Could you check a few things on this model? Use its own coordinates, in mm. A direction names the side the tool comes from. Give positions to 0.01 mm unless a question says otherwise; leave off trailing zeros. Loops run counter-clockwise (first coordinate to the right, second up) from the corner with the lowest first, then second, coordinate; pieces in that order, holes last.
1. Imagine slicing it at A-A (z = -29.5). List the corners of the cut face in (x, y) for me.
2. For faces 4 (the cylindrical face through (-0.13, 0, -30.49)), 5 (the flat face through (0, -0.25, -27)), 6 (the cylindrical face through (-1.08, -4.88, -8.87)), 7 (the flat face through (7, 1, -2)), 8 (the flat face through (0, 0.25, -27)), which set-ups out of +Z, -Z, +X, -X, +Y, -Y let a thin tool reach every point of the face, with its end or its side?
3. I need wall thicknesses on line 1 along X through (y, z) = (0.1, -29.5); line 2 along Z through (x, y) = (4.5, -1.25); line 3 along Y through (x, z) = (-3.5, -5). Which ranges of each line are inside material? Lowest first, please.
4. Imagine slicing it at C-C (z = -9). List the corners of the cut face in (x, y) for me.
5. For P1, Ø3, axis at x = 3, z = -9, coming from the -Y side; P2, Ø2.5, axis at x = 1, z = -27, coming from the -Y side; P3, Ø1.4, axis at x = -0.5, y = 4, coming from the -Z side, each with a flat end and sliding along its axis, tell me the tip position at first contact or that it passes through.
6. Thinking about a two-plate mould opening in X: for faces 1 (the flat face through (0, 0, -18)), 2 (the flat face through (2, -5, 0)), 3 (the cylindrical face through (-7.493, 0.33, -1.493)), which applies, +X half, -X half, draft (parallel to the pull), parting line (faces both ways), or undercut?
```python
from build123d import *

# Parameters (mm, degrees)
ESQUISSE1_R           = 7.5
EXTRUSION1_DEPTH      = 32
ESQUISSE2_R           = 5
ESQUISSE2_R_2         = 2.5
ESQUISSE2_R_3         = 2.45
EXTRUSION3_DEPTH      = 18
ESQUISSE3_OUTSIDE_W   = 24.678
ESQUISSE3_OUTSIDE_H   = 24.678
ESQUISSE3_OUTSIDE_R   = 6.75
EXTRUSION5_DEPTH      = 30
ESQUISSE4_OUTSIDE_W   = 24.678
ESQUISSE4_OUTSIDE_H   = 24.678
ESQUISSE4_OUTSIDE_W_2 = 5
ESQUISSE4_OUTSIDE_H_2 = 0.5
EXTRUSION6_DEPTH      = 10
ESQUISSE5_W           = 18
ESQUISSE5_H           = 6
EXTRUSION7_DEPTH      = 1
ESQUISSE6_R           = 1
EXTRUSION8_DEPTH      = 8.75
CHANFREIN1_SIZE       = 1
CHANFREIN2_SIZE       = 0.5


with BuildPart() as part:
    # Esquisse1 → Extrusion1 (new body)
    with BuildSketch(Plane.XY):
        Circle(ESQUISSE1_R)
    extrude(amount=-EXTRUSION1_DEPTH)

    # Esquisse2 → Extrusion3 (cut)
    with BuildSketch(Plane.XY):
        Circle(ESQUISSE2_R)
        Circle(ESQUISSE2_R_2, mode=Mode.SUBTRACT)
        Circle(ESQUISSE2_R_3)
    extrude(amount=-EXTRUSION3_DEPTH, mode=Mode.SUBTRACT)

    # Esquisse3 outside → Extrusion5 (cut)
    with BuildSketch(Plane(origin=(0, 0, -32), x_dir=(-1, 0, 0), z_dir=(0, 0, -1))):
        Rectangle(ESQUISSE3_OUTSIDE_W, ESQUISSE3_OUTSIDE_H)
        Circle(ESQUISSE3_OUTSIDE_R, mode=Mode.SUBTRACT)
    extrude(amount=-EXTRUSION5_DEPTH, mode=Mode.SUBTRACT)

    # Esquisse4 outside → Extrusion6 (cut)
    with BuildSketch(Plane(origin=(0, 0, -32), x_dir=(-1, 0, 0), z_dir=(0, 0, -1))):
        Rectangle(ESQUISSE4_OUTSIDE_W, ESQUISSE4_OUTSIDE_H)
        Rectangle(ESQUISSE4_OUTSIDE_W_2, ESQUISSE4_OUTSIDE_H_2, mode=Mode.SUBTRACT)
    extrude(amount=-EXTRUSION6_DEPTH, mode=Mode.SUBTRACT)

    # Esquisse5 → Extrusion7 (cut)
    with BuildSketch(Plane(origin=(0, 0, -22), x_dir=(-1, 0, 0), z_dir=(0, 0, -1))):
        with Locations((0, 5)):
            Rectangle(ESQUISSE5_W, ESQUISSE5_H)
    extrude(amount=-EXTRUSION7_DEPTH, mode=Mode.SUBTRACT)

    # Esquisse6 → Extrusion8 (cut, through all)
    with BuildSketch(Plane(origin=(0, 0.25, 0), x_dir=(1, 0, 0), z_dir=(0, 1, 0))):
        with Locations((0, 29.5)):
            Circle(ESQUISSE6_R)
    extrude(amount=-EXTRUSION8_DEPTH, mode=Mode.SUBTRACT)

    # Chanfrein1
    chanfrein1_edges = [part.edges().sort_by_distance(p)[0] for p in [
        (-7.5, 0, 0),
    ]]
    chamfer(chanfrein1_edges, length=CHANFREIN1_SIZE)

    # Chanfrein2
    chanfrein2_edges = [part.edges().sort_by_distance(p)[0] for p in [
        (1.011418624, -6.67379445, -22),
        (0, 2, -22),
    ]]
    chamfer(chanfrein2_edges, length=CHANFREIN2_SIZE)


solid = part.part
```
Derived:
1. outline: (-2.5, -0.25) - (-1, -0.25) - (-1, 0.25) - (-2.5, 0.25) - close; (1, -0.25) - (2.5, -0.25) - (2.5, 0.25) - (1, 0.25) - close
2. face 4: +Y, -Y
2. face 5: -Z, +X, -X, -Y
2. face 6: +Z
2. face 7: -Z
2. face 8: -Z, +X, -X, +Y
3. line 1: x = -2.5 to -1, 1 to 2.5
3. line 2: z = -22 to -18
3. line 3: y = -5.77 to -3.57, 3.57 to 5.77
4. outline: circle Ø13.5 at (0, 0); circle Ø5 at (0, 0); hole circle Ø10 at (0, 0); hole circle Ø4.9 at (0, 0)
5. P1: stops at y = -6.58
5. P2: stops at y = -0.25
5. P3: stops at z = -21
6. face 1: undercut
6. face 2: draft
6. face 3: parting line
